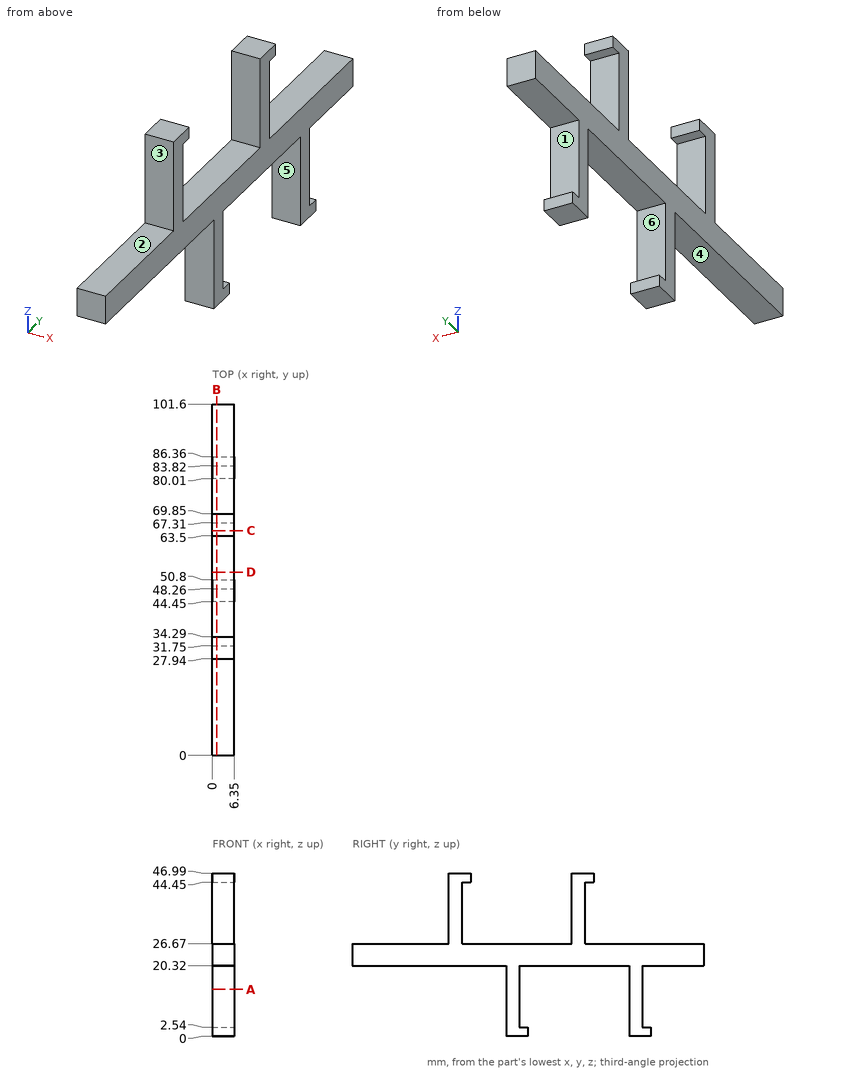
Verification items for this drawing (mm, ordinates from the low corner). A direction names the side the tool comes from. Coordinates: 2 decimals unless noted, no trailing zeros. Order: outer loops, then holes, each group sorted by start corner. A loop starts at its lowest first (then second) coordinate and runs counter-clockwise, first axis right, second up. Notation, with made-up numbers: (47.25, 34) -> (77.25, 34) arc R30 cw to (77.25, 61) -> close; hole circle Ø11 at (18, 19). An arc over 180 degrees is marked (long way). Answer as CSV lines item,"result". Start each with the question number.
1) Release check for a two-part mould opening along Z. For the marked faces 1, 2 and 3 record: released by +Z, released by -Z, zero draft, split by the parting line, or undercut.
2) Material ranges on L1, parallel to Z at x = 5.25, y = 49; L2, parallel to Y at x = 3.5, z = 7; L3, parallel to Y at x = 1, z = 38, recorded low to high. Write a range as [from, to].
3) Gauge pin test, flat ends, axial feed: pin 1 Ø3 at (x, z) = (1.5, 46.5) entering from +Y; pin 2 Ø3 at (x, z) = (1, 39.5) entering from -Y; pin 3 Ø1.9 at (x, y) = (4, 91) entering from -Z. Record the tip position at first contact, or that the pin passes through.
4) Cross-section at A-A, the plane z = 13.5. Record the boundary of the cut face in (x, y).
5) Set-up check for the marked faces 4, 5 and 6: record each of +Z, -Z, +X, -X, +Y, -Y from which the full face is reachable in a straight line by a thin tool's end or side.
6) Cross-section at D-D, the plane y = 53. Record the boundary of the cut face in (x, z).
7) Cross-section at B-B, the plane x = 1.25. Record the boundary of the cut face in (y, z), then the cut area to 3 significant figures.
8) Cross-section at C-C, the plane y = 65. Record the boundary of the cut face in (x, z).
Conclusion:
1,face 1,"undercut"
1,face 2,"released by +Z"
1,face 3,"zero draft"
2,L1,"z = [0, 2.54], [20.32, 26.67]"
2,L2,"y = [44.45, 48.26], [80.01, 83.82]"
2,L3,"y = [27.94, 31.75], [63.5, 67.31]"
3,pin 1,"stops at y = 69.85"
3,pin 2,"stops at y = 27.94"
3,pin 3,"stops at z = 20.32"
4,outline,"(0, 44.45) -> (6.35, 44.45) -> (6.35, 48.26) -> (0, 48.26) -> close; (0, 80.01) -> (6.35, 80.01) -> (6.35, 83.82) -> (0, 83.82) -> close"
5,face 4,"-Z, +X, -X, -Y"
5,face 5,"-Z, +X, -X"
5,face 6,"+X, -X"
6,outline,"(0, 20.32) -> (6.35, 20.32) -> (6.35, 26.67) -> (0, 26.67) -> close"
7,outline,"(0, 20.32) -> (44.45, 20.32) -> (44.45, 0) -> (50.8, 0) -> (50.8, 2.54) -> (48.26, 2.54) -> (48.26, 20.32) -> (80.01, 20.32) -> (80.01, 0) -> (86.36, 0) -> (86.36, 2.54) -> (83.82, 2.54) -> (83.82, 20.32) -> (101.6, 20.32) -> (101.6, 26.67) -> (67.31, 26.67) -> (67.31, 44.45) -> (69.85, 44.45) -> (69.85, 46.99) -> (63.5, 46.99) -> (63.5, 26.67) -> (31.75, 26.67) -> (31.75, 44.45) -> (34.29, 44.45) -> (34.29, 46.99) -> (27.94, 46.99) -> (27.94, 26.67) -> (0, 26.67) -> close"
7,area,"981 mm²"
8,outline,"(0, 20.32) -> (6.35, 20.32) -> (6.35, 46.99) -> (0, 46.99) -> close"
